Study the drawing (mm; zero at the part's minimum x, y, z) and answer. Give positions to 0.01 mm unless a question says otherwise; leave off trailing zeros. Loops run counter-clockwise (first coordinate to the right, second up) from the corner with the lowest first, then second, coordinate; pieces in that order, holes last. Notation, with made-up numbers: (54.25, 74) - (106.25, 74) arc R27 ccw to (106.25, 101) - close; hole circle Ø6 at (32, 40). An arc over 180 degrees is marked (long way). One line per item, written item: value. Start each with the question number.
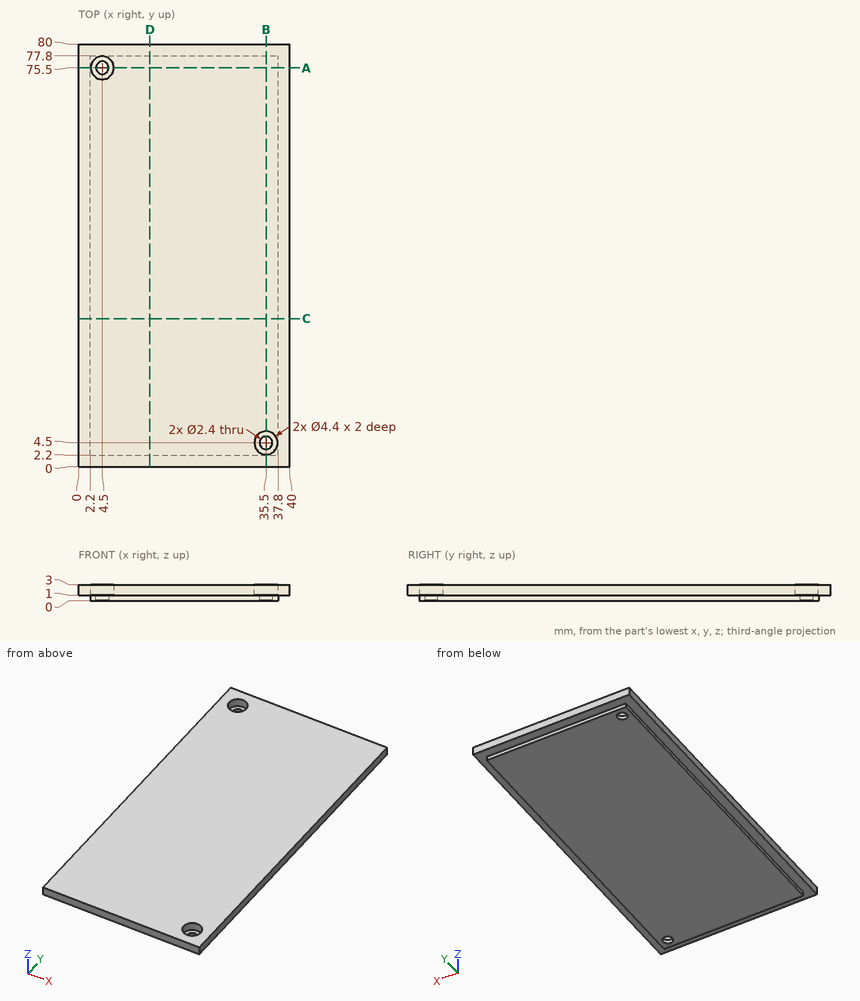
1. A cutting plane is placed at C-C (y = 28). Determine the outline of the cut face in (x, z), plus the area to 3 significant figures.
2. A cutting plane is placed at D-D (x = 13.5). Determine the outline of the cut face in (y, z), plus the area to 3 significant figures.
3. Flat-ended cylindrical pins translate along their axes: pin 1 (3.5 mm diameter, centred on x = 35.5, y = 4.5, fed in from -Z); pin 2 (2 mm diameter, centred on x = 35.5, y = 4.5, fed in from -Z); pin 3 (3.5 mm diameter, centred on x = 4.5, y = 75.5, fed in from +Z); pin 4 (0.5 mm diameter, centred on x = 25.5, z = 0.5, fed in from +Y). Find the tip coordinate at first contact, or state that the pin passes through.
4. A cutting plane is placed at A-A (y = 75.5). Determine the outline of the cut face in (x, z), plus the area to 3 significant figures.
5. Find the intervals of material crossed by L1, parallel to X at y = 75.5, z = 0.5; L2, parallel to Y at x = 35.5, z = 0.45; L3, parallel to Y at x = 35.5, z = 1.45, in increasing order. Write a range as [from, to].
6. A cutting plane is placed at B-B (x = 35.5). Determine the outline of the cut face in (y, z).
Results below:
1. outline: (0, 1) - (2.2, 1) - (2.2, 0) - (37.8, 0) - (37.8, 1) - (40, 1) - (40, 3) - (0, 3) - close
1. area: 116 mm^2
2. outline: (0, 1) - (2.2, 1) - (2.2, 0) - (77.8, 0) - (77.8, 1) - (80, 1) - (80, 3) - (0, 3) - close
2. area: 236 mm^2
3. pin 1: stops at z = 0
3. pin 2: passes through
3. pin 3: stops at z = 1
3. pin 4: stops at y = 77.8
4. outline: (0, 1) - (2.2, 1) - (2.2, 0) - (3.3, 0) - (3.3, 1) - (2.3, 1) - (2.3, 3) - (0, 3) - close; (5.7, 0) - (37.8, 0) - (37.8, 1) - (40, 1) - (40, 3) - (6.7, 3) - (6.7, 1) - (5.7, 1) - close
4. area: 104 mm^2
5. L1: x = [2.2, 3.3], [5.7, 37.8]
5. L2: y = [2.2, 3.3], [5.7, 77.8]
5. L3: y = [0, 2.3], [6.7, 80]
6. outline: (0, 1) - (2.2, 1) - (2.2, 0) - (3.3, 0) - (3.3, 1) - (2.3, 1) - (2.3, 3) - (0, 3) - close; (5.7, 0) - (77.8, 0) - (77.8, 1) - (80, 1) - (80, 3) - (6.7, 3) - (6.7, 1) - (5.7, 1) - close
